Work out the finished part from the listing and answer in its coordinate system (mm). A direction names the side the tool comes from. Round coordinates to 2 decimals unless told otherwise and drop trailing zeros. Order: outer loops, then holes, each group sorted by start corner. A loop starts at its lowest first (then second) coordinate and runs counter-clockwise, first axis right, second up. Notation, with made-up numbers: (6, 48.5) - (36, 48.5) arc R22 cw to (36, 73.5) - close; hole circle Ø7 at (66.25, 64). An arc over 180 degrees is marked (long way). Answer in a Markdown table with one row per item.
from build123d import *

# Parameters (mm, degrees)
SKETCH1_R           = 6.2865
BASE_EXTRUDE_DEPTH  = 40
SKETCH3_R           = 9.4615
BOSS_EXTRUDE1_DEPTH = 15.875
SKETCH4_R           = 6.35
CUT_EXTRUDE1_DEPTH  = 12.7
FILLET1_R           = 4.7625
FILLET2_R           = 4.7625
CUT_EXTRUDE3_START  = -6.35
CUT_EXTRUDE3_DEPTH  = 6.35
CHAMFER1_SIZE       = 0.79375


with BuildPart() as part:
    # Sketch1 → Base-Extrude (new body)
    with BuildSketch(Plane(origin=(0, 0, 0), x_dir=(-1, 0, 0), z_dir=(0, 1, 0))):
        with Locations(Location((0, 0, 0), (0, 0, 90))):
            Circle(SKETCH1_R)
    extrude(amount=BASE_EXTRUDE_DEPTH)

    # Sketch3 → Boss-Extrude1 (add)
    with BuildSketch(Plane(origin=(0, 0, 0), x_dir=(-1, 0, 0), z_dir=(0, 1, 0))):
        with Locations(Location((0, 0, 0), (0, 0, 90))):
            Circle(SKETCH3_R)
    extrude(amount=BOSS_EXTRUDE1_DEPTH)

    # Sketch4 → Cut-Extrude1 (cut)
    with BuildSketch(Plane(origin=(0, 0, 0), x_dir=(-1, 0, 0), z_dir=(0, 1, 0))):
        with Locations(Location((0, 0, 0), (0, 0, 90))):
            Circle(SKETCH4_R)
    extrude(amount=CUT_EXTRUDE1_DEPTH, mode=Mode.SUBTRACT)

    # Fillet1
    # the kernel refuses this fillet: 4.7625 mm, written as the material it adds along each edge
    with BuildSketch(Plane(origin=(0, 15.875, 0), x_dir=(0, 0, 1), z_dir=(1, 0, 0))) as fillet1_piece_1:
        with BuildLine():
            CenterArc((11.049, -4.490128061), FILLET1_R, 109.471220634, 70.528779366)
            Line((6.2865, -4.490128061), (6.19125, -4.490128061))
            Line((6.19125, -4.490128061), (6.19125, 0))
            Line((6.19125, 0), (6.2865, 0.09525))
            ThreePointArc((6.2865, 0.09525), (7.874, 0.09525), (9.42975, 0.089802561))
            Line((9.42975, 0.089802561), (9.4615, 0))
        make_face()
    revolve(axis=Axis((0, 15.875, 0), (0, -1, 0)))

    # Fillet2
    fillet2_edges = [part.edges().sort_by_distance(p)[0] for p in [
        (0, 15.875, -9.4615),
    ]]
    fillet(fillet2_edges, radius=FILLET2_R)

    # Sketch7 → Cut-Extrude3 (cut)
    with BuildSketch(Plane(origin=(0, 40, 0), x_dir=(-1, 0, 0), z_dir=(0, 1, 0)).offset(CUT_EXTRUDE3_START)):
        with BuildLine():
            Line((-4.8895, 3.951312693), (-4.8895, -3.951312693))
            ThreePointArc((-4.8895, -3.951312693), (-6.2865, 0), (-4.8895, 3.951312693))
        make_face()
    extrude(amount=CUT_EXTRUDE3_DEPTH, mode=Mode.SUBTRACT)

    # Chamfer1
    chamfer1_edges = [part.edges().sort_by_distance(p)[0] for p in [
        (-5.67274226, 40, -2.70925774),
    ]]
    chamfer(chamfer1_edges, length=CHAMFER1_SIZE)


solid = part.part
1) Find the intervals of material crossed by probe 1 along X at (y, z) = (8.75, 0); probe 2 along Z at (x, y) = (-0.75, 11.5); probe 3 along Y at (x, z) = (-3, 2), in increasing order. Write a range as from..to.
Filled in:
| item | result |
|---|---|
| probe 1 | x = -9.46..-6.35, 6.35..9.46 |
| probe 2 | z = -9.43..-6.31, 6.31..9.43 |
| probe 3 | y = 12.7..40 |
2) Find section B-B, the plane y = 33. Give the vertices of the cut face in (x, z), then the cut area to 3 significant figures.
Filled in:
| item | result |
|---|---|
| outline | circle Ø12.57 at (0, 0) |
| area | 124 mm^2 |
3) Each of these flat-tipped pins is pushed along its axis until it touches: pin 1 (3 mm diameter, centred on y = 5, z = -3.5, fed in from -X); pin 2 (10 mm diameter, centred on x = -2.5, z = -2.5, fed in from -Y); pin 3 (1.5 mm diameter, centred on x = -7.5, y = 29, fed in from -Z); pin 4 (4 mm diameter, centred on y = 34.5, z = 6, fed in from -X). Where does it stop, or does it pass through?
Filled in:
| item | result |
|---|---|
| pin 1 | stops at x = -9.25 |
| pin 2 | stops at y = 0 |
| pin 3 | passes through |
| pin 4 | stops at x = -4.85 |
4) Which of the six approach directions +Z, -Z, +X, -X, +Y, -Y give full straight-line access (tool end or side, diameter ignored) to faces 1 (the face through (-5.62, 39.87, -0.21)), 2 (the face through (4.89, 37, 0)), 3 (the face through (0, 12.7, 0))?
Filled in:
| item | result |
|---|---|
| face 1 | +Y |
| face 2 | +Z, -Z, +X, +Y |
| face 3 | -Y |
5) The mould has two halves that part along Z. Classify faces 4 (the face through (0, 40, 0)), 5 (the face through (-3.86, 6.26, -5.04)), 6 (the face through (-6.137, 29.654, -1.363)): released by +Z, released by -Z, zero draft, split by the parting line, or undercut.
Filled in:
| item | result |
|---|---|
| face 4 | zero draft |
| face 5 | undercut |
| face 6 | split by the parting line |
6) Find section A-A, the plane y = 3. Give the vertices of the cut face in (x, z), then the cut area to 3 significant figures.
Filled in:
| item | result |
|---|---|
| outline | circle Ø18.92 at (0, 0); hole circle Ø12.7 at (0, 0) |
| area | 155 mm^2 |
